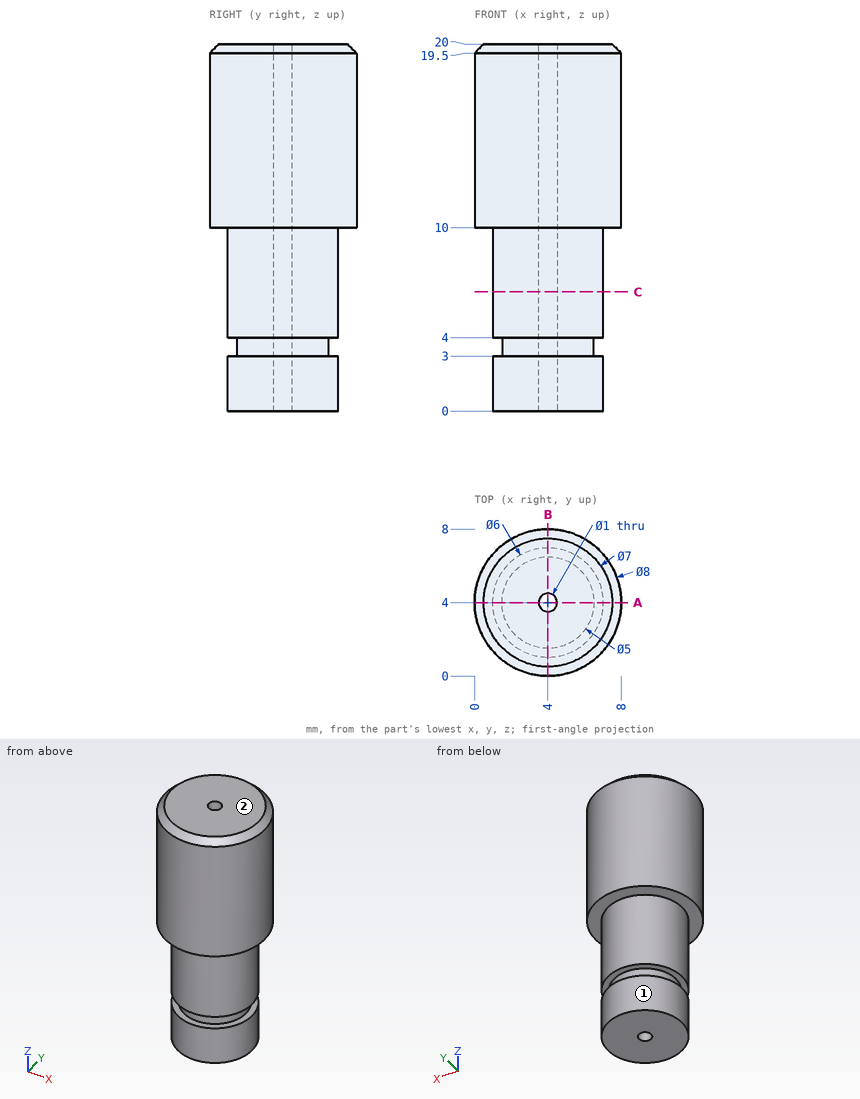
Study the drawing (mm; zero at the part's minimum x, y, z) and answer. A direction names the side the tool comes from. Round coordinates to 2 decimals unless told otherwise and drop trailing zeros. Write each loop counter-clockwise with the first axis right and the second up, starting at its lowest first coordinate (ties: lowest second). Pieces come first, ordered by that corner, then holes. Notation, with made-up numbers: (67.25, 1.5) - (126.25, 1.5) arc R27 cw to (126.25, 18.5) - close; hole circle Ø8 at (8, -21.75). An arc over 180 degrees is marked (long way). Use a Markdown table: item, result. Add a question column.
1. Flat-ended cylindrical pins translate along their axes: P1, Ø1.5, axis at y = 5, z = 13, coming from the +X side; P2, Ø1.5, axis at y = 4, z = 2.5, coming from the +X side. Find the tip coordinate at first contact, or state that the pin passes through.
2. Consider line 1 (Y direction, x = 4, z = 12.75); line 2 (Z direction, x = 5.5, y = 1.5); line 3 (Y direction, x = 4, z = 5.5). Determine where each line is inside the solid, lowest interval first.
3. A tool of negligible diameter and unlimited length cuts with its end or side. For the marked faces 1 and 2, from which of +Z, -Z, +X, -X, +Y, -Y can it reach the whole face along a straight path? Write none if from no direction.
4. The part is cut by section A-A (y = 4). Write down the section's boundary in (x, z).
5. The part is cut by section C-C (z = 6.5). Write down the section's boundary in (x, y).
Reported:
| question | item | result |
|---|---|---|
| 1 | P1 | x = 7.99 |
| 1 | P2 | x = 7 |
| 2 | line 1 | 0 to 3.5, 4.5 to 8 |
| 2 | line 2 | 0 to 3, 4 to 20 |
| 2 | line 3 | 1 to 3.5, 4.5 to 7 |
| 3 | face 1 | -Z |
| 3 | face 2 | +Z, +X, -X, +Y, -Y |
| 4 | outline | (0, 10) - (1, 10) - (1, 4) - (1.5, 4) - (1.5, 3) - (1, 3) - (1, 0) - (3.5, 0) - (3.5, 20) - (0.5, 20) - (0, 19.5) - close; (4.5, 0) - (7, 0) - (7, 3) - (6.5, 3) - (6.5, 4) - (7, 4) - (7, 10) - (8, 10) - (8, 19.5) - (7.5, 20) - (4.5, 20) - close |
| 5 | outline | circle Ø6 at (4, 4); hole circle Ø1 at (4, 4) |
